Check sheet for the modelled part. Datum: model origin and axes. Units: mm. A direction names the side the tool comes from. Give positions to 0.01 mm unless a question says otherwise; leave off trailing zeros. Loops run counter-clockwise (first coordinate to the right, second up) from the corner with the lowest first, then second, coordinate; pieces in that order, holes last. Notation, with made-up numbers: (-33.5, -34.75) -> (-14.5, -34.75) arc R11 cw to (-14.5, -30.75) -> close; hole circle Ø9 at (75.25, 0). An arc over 180 degrees is marked (long way). Answer as CSV lines item,"result". Start each with the question number.
(1) Gauge pin test, flat ends, axial feed: pin 1 Ø3 at (x, z) = (5.5, 11.5) entering from -Y; pin 2 Ø6.5 at (x, y) = (12, 7.5) entering from -Z; pin 3 Ø4.5 at (x, y) = (-14, 5.125) entering from -Z. Record the tip position at first contact, or that the pin passes through.
(2) Release check for a two-part mould opening along X. For faces 6 (the face through (-0.127, 9.86, 0.154)), 7 (the face through (0, 20, 6)), 8 (the face through (12.43, 5.78, 9.08)) record: pulls with the +X half, pulls with the -X half, needs draft (parallel to the pull), parting line crosses it, or undercut.
(3) Section check A-A on z = 9.5. Enter the section's corners in (x, y) (3 decimals), plus the area to 3 significant figures.
(4) Section check D-D on z = 7.5. Enter the section's corners in (x, y) (3 decimals).
(5) Material ranges on line 1 (Y direction, x = 14, z = 7.5) (3 decimals); line 2 (Y direction, x = -14, z = 6) (3 decimals); line 3 (X direction, y = 10, z = 14.75), recorded low to high. Write a range as from..to.
(6) Access from +Z, -Z, +X, -X, +Y, -Y to the whole of each face (thin tool, end or side, straight path). Record for faces 1 (the face through (-13, 10, 3)), 2 (the face through (-15.62, 14.61, 9.08)), 3 (the face through (13, 10, 3)), 4 (the face through (-15.25, 10, 11)), 5 (the face through (13, 12, 15)).
(7) Section check B-B on x = -13. Enter the section's corners in (y, z).
Autodesk Fusion 360 part; units mm, degrees
sketch "スケッチ1" plane through (0, 0, 0) normal (0, 0, 1) x (1, 0, 0)
  line L0 (-19, 20) -> (19, 20)
  line L1 (19, 20) -> (19, 0)
  line L2 (19, 0) -> (-19, 0)
  line L3 (-19, 0) -> (-19, 20)
  dimension "d1" = 38
  dimension "d2" = 20
extrude "押し出し1" add sketch "スケッチ1" along normal blind 15
sketch "スケッチ2" plane through (0, 0, 0) normal (0, -1, 0) x (1, 0, 0)
  line L0 (-19, 0) -> (19, 0)
  line L1 (19, 0) -> (19, 15)
  line L2 (19, 15) -> (-19, 15)
  line L3 (-19, 15) -> (-19, 0)
  line L4 (-19, 15.1531) -> (19, 15.1531) construction
  arc A0 (-8.5, 15.1531) -> (8.5, 15.1531) centre (0, 15.1531) ccw
  line L5 (8.5, 15.1531) -> (8.5, 15)
  line L6 (-8.5, 15.1531) -> (-8.5, 15)
  dimension "d6" = 17
extrude "押し出し2" cut sketch "スケッチ2" against normal blind 20 contours L2 A0
ref_plane "WorkPlane2" through (0, 10, 0) normal (0, 1, 0) x (0, 0, 1)
sketch "Sketch5" plane through (0, 10, 0) normal (0, 1, 0) x (1, 0, 0)
  line L0 (15.25, -15) -> (0, -15)
  line L1 (15.25, -7) -> (15.25, -15)
  line L2 (0, -5) -> (15.25, -7)
  arc A0 (3.3966, -15) -> (-3.3966, -15) centre (0, -15.1531) ccw
  line L3 (3.3966, -15) -> (19, -15)
  line L4 (19, -15) -> (19, 0)
  line L5 (19, 0) -> (-19, 0)
  line L6 (-19, 0) -> (-19, -15)
  line L7 (-19, -15) -> (-3.3966, -15)
  line L8 (-15.25, -15) -> (0, -15)
  line L9 (-15.25, -7) -> (-15.25, -15)
  line L10 (0, -5) -> (-15.25, -7)
extrude "Extrude5" cut sketch "Sketch5" along normal blind 0.85 and the other way blind 0.85 contours L0 L1 L2 A0 L3 L7 L8 L9 L10
sketch "スケッチ4" plane through (0, 0, 15) normal (0, 0, 1) x (-1, 0, 0)
  line L0 (8.4986, -20) -> (19, -20)
  line L1 (19, -20) -> (19, 0)
  line L2 (19, 0) -> (8.4986, 0)
  line L3 (19, -15.125) -> (-17.5478, -15.125) construction
  line L4 (-19, -20) -> (-8.4986, -20) construction
  line L5 (19, -5.125) -> (-19, -5.125) construction
  line L6 (-19, 0) -> (-19, -20) construction
  circle A0 centre (-14, -15.125) radius 1.7
  circle A1 centre (-14, -5.125) radius 1.7
  circle A2 centre (14, -15.125) radius 1.7
  circle A3 centre (14, -5.125) radius 1.7
  line L7 (15.25, -10.85) -> (8.4986, -10.85)
  line L8 (8.4986, -10.85) -> (8.4986, -20)
  line L9 (8.4986, 0) -> (8.4986, -9.15)
  line L10 (8.4986, -9.15) -> (15.25, -9.15)
  line L11 (15.25, -9.15) -> (15.25, -10.85)
  dimension "d15" = 4.875
  dimension "d16" = 10
  dimension "d17" = 3.4
  dimension "d18" = 5
  dimension "d19" = 3.4
  dimension "d20" = 5
  dimension "d21" = 3.4
  dimension "d22" = 5
  dimension "d23" = 3.4
  dimension "d24" = 5
extrude "押し出し4" cut sketch "スケッチ4" against normal blind 25 contours A0 | A1 | A2 | A3
sketch "Sketch6" plane through (0, 0, 0) normal (0, -1, 0) x (1, 0, 0)
  arc A0 (-8.4986, 15) -> (8.4986, 15) centre (0, 15.1531) ccw
  line L0 (-8.4986, 15) -> (-19, 15)
  line L1 (-19, 15) -> (-19, 0)
  line L2 (-19, 0) -> (19, 0)
  line L3 (19, 0) -> (19, 15)
  line L4 (19, 15) -> (8.4986, 15)
  circle A1 centre (0, 15.1531) radius 15
  line L5 (-19, 15) -> (19, 15)
  line L6 (19, 15) -> (19, 3)
  line L7 (19, 3) -> (-19, 3)
  line L8 (-19, 3) -> (-19, 15)
  dimension "d32" = 30
  dimension "d33" = 12
extrude "Extrude6" cut sketch "Sketch6" against normal blind 25 contours L1 L2 L3 A1 L7
fillet "Fillet1" radius 1 2 edges at (-8.7921, 10, 3) (8.7921, 10, 3)
move_face "OffsetFaces1" offset -1.5 1 faces at (-19, 6.6667, 7)
move_face "OffsetFaces2" offset -1.5 1 faces at (19, 13.3333, 7)
Working result:
1,pin 1,"passes through"
1,pin 2,"stops at z = 2.93"
1,pin 3,"stops at z = 3"
2,face 6,"parting line crosses it"
2,face 7,"needs draft"
2,face 8,"undercut"
3,outline,"(-17.5, 0) -> (-6.348, 0) -> (-6.348, 9.15) -> (-15.25, 9.15) -> (-15.25, 10.85) -> (-6.348, 10.85) -> (-6.348, 20) -> (-17.5, 20) -> close; (6.348, 0) -> (17.5, 0) -> (17.5, 20) -> (6.348, 20) -> (6.348, 10.85) -> (15.25, 10.85) -> (15.25, 9.15) -> (6.348, 9.15) -> close; hole circle Ø3.4 at (-14, 5.125); hole circle Ø3.4 at (-14, 15.125); hole circle Ø3.4 at (14, 5.125); hole circle Ø3.4 at (14, 15.125)"
3,area,"380 mm^2"
4,outline,"(-17.5, 0) -> (-3.699, 0) -> (-3.699, 9.15) -> (-15.25, 9.15) -> (-15.25, 10.85) -> (-3.699, 10.85) -> (-3.699, 20) -> (-17.5, 20) -> close; (3.699, 0) -> (17.5, 0) -> (17.5, 20) -> (3.699, 20) -> (3.699, 10.85) -> (15.25, 10.85) -> (15.25, 9.15) -> (3.699, 9.15) -> close; hole circle Ø3.4 at (-14, 5.125); hole circle Ø3.4 at (-14, 15.125); hole circle Ø3.4 at (14, 5.125); hole circle Ø3.4 at (14, 15.125)"
5,line 1,"y = 0..3.425, 6.825..9.15, 10.85..13.425, 16.825..20"
5,line 2,"y = 0..3.425, 6.825..13.425, 16.825..20"
5,line 3,"x = -17.5..-15.25, 15.25..17.5"
6,face 1,"-Z, -X, +Y, -Y"
6,face 2,"+Z, -Z"
6,face 3,"-Z, +X, +Y, -Y"
6,face 4,"+Z"
6,face 5,"+Z, +X, -X, +Y, -Y"
7,outline,"(0, 3) -> (3.75, 3) -> (3.75, 15) -> (0, 15) -> close; (6.5, 3) -> (13.75, 3) -> (13.75, 15) -> (10.85, 15) -> (10.85, 6.7) -> (9.15, 6.7) -> (9.15, 15) -> (6.5, 15) -> close; (16.5, 3) -> (20, 3) -> (20, 15) -> (16.5, 15) -> close"
